Part model, mm, in its own coordinate system. A direction names the side the tool comes from. Coordinates: 2 decimals unless noted, no trailing zeros. Loops run counter-clockwise (first coordinate to the right, second up) from the corner with the lowest first, then second, coordinate; pieces in that order, holes last. Notation, with made-up numbers: M 34,89 L 66,89 A21 cw 66,116 Z; hole C -17.75,85.5 d8. An arc over 180 degrees is marked long. Use CSV: the item, a comma, the result in double quotes. Start each with the question number.
from build123d import *

# Parameters (mm, degrees)
SKETCH_1_R      = 4
SKETCH_1_R_2    = 2
EXTRUDE_1_DEPTH = 1.5


with BuildPart() as part:
    # 草图1 → 凸台-拉伸1 (new, symmetric)
    with BuildSketch(Plane.XY):
        with BuildLine():
            Line((5.590169944, 5), (49.5, 5))
            ThreePointArc((49.5, 5), (54.5, 0), (49.5, -5))
            Line((49.5, -5), (5.590169944, -5))
            ThreePointArc((5.590169944, -5), (-7.5, 0), (5.590169944, 5))
        make_face()
        Circle(SKETCH_1_R, mode=Mode.SUBTRACT)
        with Locations((49.5, 0)):
            Circle(SKETCH_1_R_2, mode=Mode.SUBTRACT)
        with BuildLine():
            Line((11, 1), (14, 1))
            ThreePointArc((14, 1), (15, 0), (14, -1))
            Line((14, -1), (11, -1))
            ThreePointArc((11, -1), (10, 0), (11, 1))
        make_face(mode=Mode.SUBTRACT)
    extrude(amount=EXTRUDE_1_DEPTH, both=True)


solid = part.part
1. Wall check: probe 1 along Y at (x, z) = (49.5, -0.1); probe 2 along X at (y, z) = (0.25, 0.05); probe 3 along X at (y, z) = (-1.25, 0.9). Give the ranges that are in metal, low to high.
2. Pin check, flat tips, straight feed: pin 1 (0.9 mm diameter, centred on x = 12, z = 0, fed in from -Y); pin 2 (1.5 mm diameter, centred on x = 13, z = -0.5, fed in from +Y); pin 3 (3 mm diameter, centred on x = 49.5, y = 0, fed in from -Z). Stop position of each tip, or through.
3. Slice it at D-D, the plane x = 0. List the corners of the cut face in (y, z), and give its area (3 significant figures).
4. Slice it at B-B, the plane z = -0.85. List the corners of the cut face in (x, y), and give its area (3 significant figures).
5. Slice it at C-C, the plane x = 12.5. List the corners of the cut face in (y, z).
6. Tool access for faces 1 (the face through (13, -1, 0)), 2 (the face through (28, -5, 0)), 3 (the face through (27, 5, 0)): list every direction of +Z, -Z, +X, -X, +Y, -Y with a clear straight run to the whole face (end or side of a thin tool).
7. Slice it at A-A, the plane y = 0. List the corners of the cut face in (x, z), and give its area (3 significant figures).
8. Two-plate mould, pull along Y, no slides. Class faces 4 (the face through (24, -2, -1.5)), 5 (the face through (10, 0, 0)), 6 (the face through (-7.496, -0.253, 0.021)): pulls with the +Y half, pulls with the -Y half, needs draft (parallel to the pull), parting line crosses it, or undercut.
Found:
1,probe 1,"-5 to -2, 2 to 5"
1,probe 2,"-7.5 to -3.99, 3.99 to 10.03, 14.97 to 47.52, 51.48 to 54.49"
1,probe 3,"-7.4 to -3.8, 3.8 to 47.94, 51.06 to 54.34"
2,pin 1,"y = -5"
2,pin 2,"y = 5"
2,pin 3,"through"
3,outline,"M -7.5,-1.5 L -4,-1.5 L -4,1.5 L -7.5,1.5 Z; M 4,-1.5 L 7.5,-1.5 L 7.5,1.5 L 4,1.5 Z"
3,area,"21.0 mm^2"
4,outline,"M 5.59,-5 L 49.5,-5 A5 ccw 49.5,5 L 5.59,5 A7.5 ccw long Z; hole C 0,0 d8; hole M 11,-1 L 14,-1 A1 ccw 14,1 L 11,1 A1 ccw Z; hole C 49.5,0 d4"
4,area,"570 mm^2"
5,outline,"M -5,-1.5 L -1,-1.5 L -1,1.5 L -5,1.5 Z; M 1,-1.5 L 5,-1.5 L 5,1.5 L 1,1.5 Z"
6,face 1,"+Z, -Z"
6,face 2,"+Z, -Z, +X, -Y"
6,face 3,"+Z, -Z, +X, +Y"
7,outline,"M -7.5,-1.5 L -4,-1.5 L -4,1.5 L -7.5,1.5 Z; M 4,-1.5 L 10,-1.5 L 10,1.5 L 4,1.5 Z; M 15,-1.5 L 47.5,-1.5 L 47.5,1.5 L 15,1.5 Z; M 51.5,-1.5 L 54.5,-1.5 L 54.5,1.5 L 51.5,1.5 Z"
7,area,"135 mm^2"
8,face 4,"needs draft"
8,face 5,"undercut"
8,face 6,"parting line crosses it"
